Geometry check sheet. Reference: drawing and pictorial views, mm from the part's lowest x, y, z. A direction names the side the tool comes from. Round coordinates to 2 decimals unless told otherwise and drop trailing zeros. Write each loop counter-clockwise with the first axis right and the second up, starting at its lowest first coordinate (ties: lowest second). Pieces come first, ordered by that corner, then holes. Notation, with made-up numbers: (46.25, 28) - (51.25, 28) arc R24 ccw to (51.25, 64) - close; hole circle Ø1 at (15.5, 23.5). An arc over 180 degrees is marked (long way). Use one line per item in the form item = value. Start each with the question number.
1) Section check B-B (z = 8.5). Count the separate pieces of the cut face and the enclosed holes in it, then the cut area to 3 significant figures.
2) Section check D-D (z = 56.5). Record the boundary of the cut face in (x, y) (1 decimal), then the cut area to 3 significant figures.
3) Scan lines: probe 1 along Y at (x, z) = (61.5, 19); probe 2 along Z at (x, y) = (152, 91). Record each from-to range of solid material in increasing order.
4) Set-up check for the marked faces 1 and 2: record each of +Z, -Z, +X, -X, +Y, -Y from which the full face is reachable in a straight line by a thin tool's end or side.
5) Draft check along Y on the marked faces 3, 4 and 5. Enter one of: +Y half, -Y half, draft (parallel to the pull), parting line (faces both ways), or undercut.
6) Gauge pin test, flat ends, axial feed: P1, Ø2.5, axis at y = 6, z = 10.5, coming from the -X side (1 decimal); P2, Ø10, axis at y = 47, z = 27.5, coming from the +X side; P3, Ø8, axis at x = 145.5, z = 23, coming from the +Y side (1 decimal); P4, Ø2.5, axis at x = 158.5, z = 10, coming from the -Y side (1 decimal). Record the tip position at first contact, or that the pin passes through.
7) Section check A-A (x = 91.5). Record the boundary of the cut face in (y, z), then the cut area to 3 significant figures.
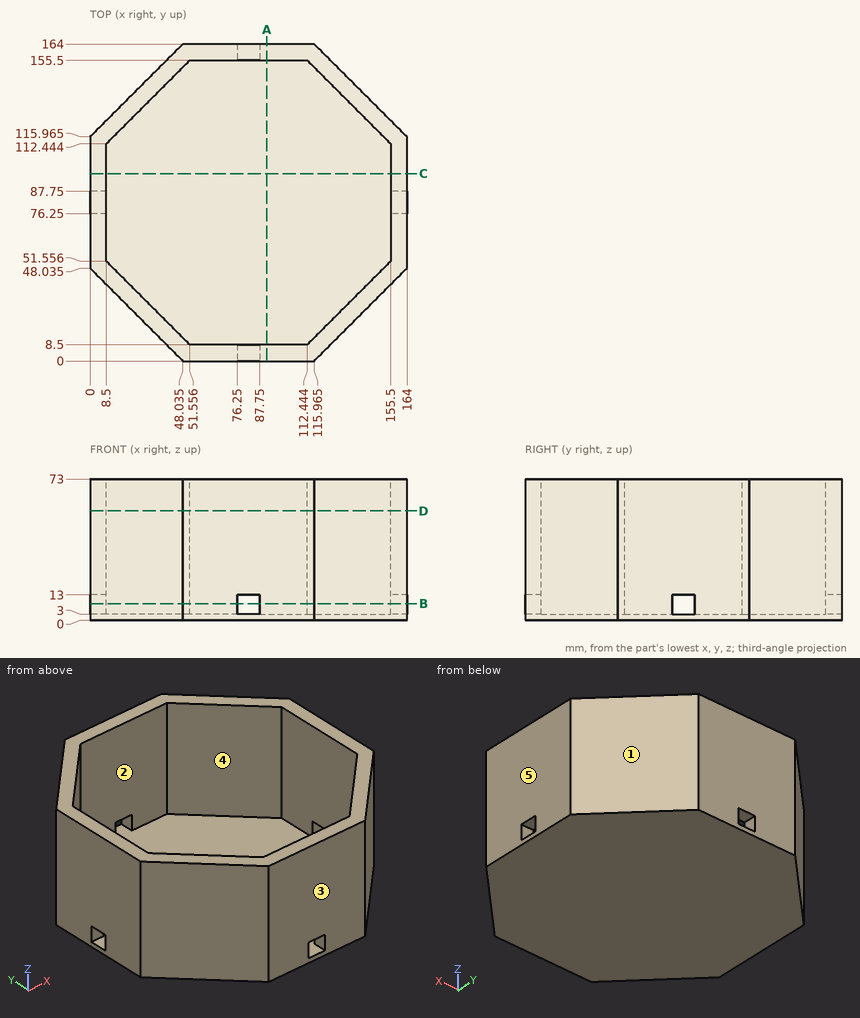
Results are:
q1.separate_pieces = 4
q1.enclosed_holes = 0
q1.area = 3,990 mm²
q2.outline = (0, 48) - (48, 0) - (116, 0) - (164, 48) - (164, 116) - (116, 164) - (48, 164) - (0, 116) - close; hole (8.5, 51.6) - (51.6, 8.5) - (112.4, 8.5) - (155.5, 51.6) - (155.5, 112.4) - (112.4, 155.5) - (51.6, 155.5) - (8.5, 112.4) - close
q2.area = 4,380 mm²
q3.probe_1 = 0 to 8.5, 155.5 to 164
q3.probe_2 = 0 to 3
q4.face_1 = +Z, -Z, +X, +Y
q4.face_2 = +Z
q5.face_3 = -Y half
q5.face_4 = undercut
q5.face_5 = draft
q6.P1 = 40.8
q6.P2 = 164
q6.P3 = 138.5
q6.P4 = 41.3
q7.outline = (0, 0) - (164, 0) - (164, 73) - (155.5, 73) - (155.5, 3) - (8.5, 3) - (8.5, 73) - (0, 73) - close
q7.area = 1,680 mm²
